Here's the drawing with two shaded views (mm, measured from the low corner). I have some questions. Round coordinates to 2 decimals unless told otherwise and drop trailing zeros. Loops run counter-clockwise (first coordinate to the right, second up) from the corner with the lowest first, then second, coordinate; pieces in that order, holes last. Notation, with made-up numbers: (37, -27.75) -> (59, -27.75) arc R32 ccw to (59, 9.25) -> close; hole circle Ø9 at (87, 37). An arc over 180 degrees is marked (long way). One line per item, written item: value. Start each with the question number.
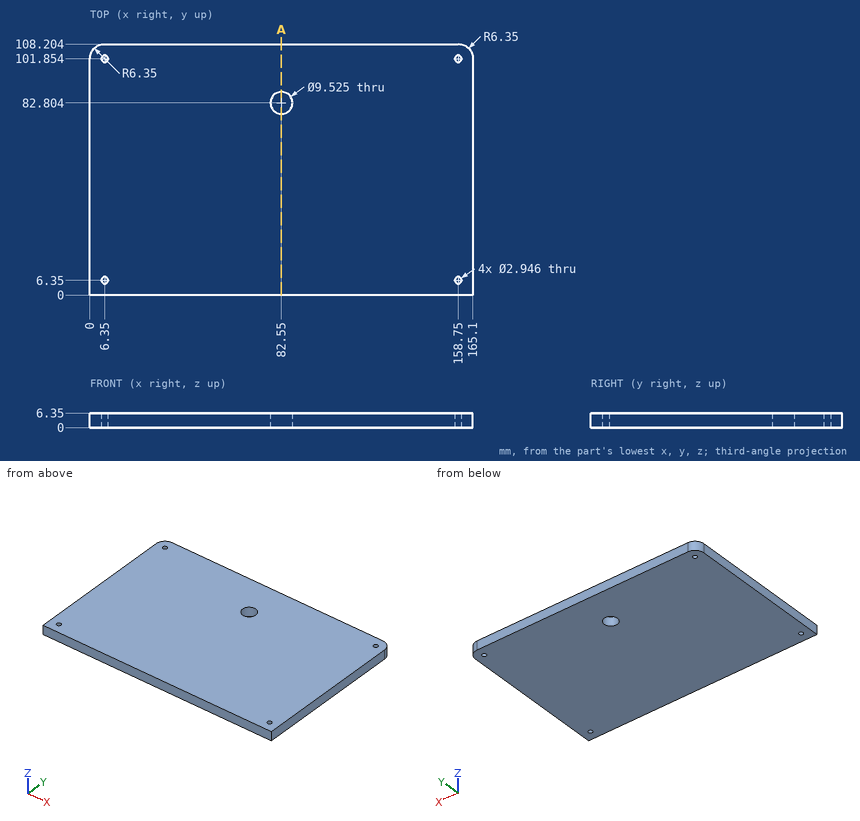
Q1. If I drill on line 1 along Y through (x, z) = (6.35, 2); line 2 along Y through (x, z) = (82.55, 2), over which ranges is the centre line in solid material (lowest first)?
Q2. Will these pins go through, and if not, where does the flat tip stop? P1, Ø2.5, axis at x = 6.35, y = 6.35, coming from the +Z side; P2, Ø4, axis at x = 158.75, y = 6.35, coming from the -Z side.
Q3. I want a section at A-A on x = 82.55. Please give me the cut outline in (y, z).
Answers below:
1. line 1: y = 0 to 4.88, 7.82 to 100.38, 103.33 to 108.2
1. line 2: y = 0 to 78.04, 87.57 to 108.2
2. P1: passes through
2. P2: stops at z = 0
3. outline: (0, 0) -> (78.04, 0) -> (78.04, 6.35) -> (0, 6.35) -> close; (87.57, 0) -> (108.2, 0) -> (108.2, 6.35) -> (87.57, 6.35) -> close
